Read the model definition and answer for the solid it produces. Units are mm, in the model's axes. A direction names the side the tool comes from. Give positions to 0.01 mm unless a question says otherwise; leave off trailing zeros. Order: outer loops, then holes, each group sorted by start corner. A loop starts at its lowest first (then second) coordinate and runs counter-clockwise, first axis right, second up. Notation, with made-up numbers: (-22.5, -9) - (11.5, -9) arc R28 ccw to (11.5, 16) - close; hole circle Ø11 at (-27, 21). An arc over 180 degrees is marked (long way). Return JSON: item names as keys, results as strings.
```python
from build123d import *

# Parameters (mm, degrees)
SKIZZE1_R                       = 30.405
SKIZZE1_R_2                     = 28.405
AUFSATZ_LINEAR_AUSTRAGEN1_DEPTH = 10
SKIZZE2_R                       = 30.405
AUFSATZ_LINEAR_AUSTRAGEN2_DEPTH = 1
AUFSATZ_LINEAR_START            = 10
AUFSATZ_LINEAR_AUSTRAGEN3_DEPTH = 10
SKIZZE5_R                       = 1.5
SCHNITT_LINEAR_AUSTRAGEN2_DEPTH = 10
SKIZZE6_W                       = 6
SKIZZE6_H                       = 10
SCHNITT_LINEAR_AUSTRAGEN3_DEPTH = 10


with BuildPart() as part:
    # Skizze1 → Aufsatz-Linear austragen1 (new body)
    with BuildSketch(Plane(origin=(0, 0, 0), x_dir=(1, 0, 0), z_dir=(0, 1, 0))):
        with Locations(Location((0, 0, 0), (0, 0, 270))):
            Circle(SKIZZE1_R)
        with Locations(Location((0, 0, 0), (0, 0, 270))):
            Circle(SKIZZE1_R_2, mode=Mode.SUBTRACT)
    extrude(amount=AUFSATZ_LINEAR_AUSTRAGEN1_DEPTH)

    # Skizze2 → Aufsatz-Linear austragen2 (add)
    with BuildSketch(Plane(origin=(0, 10, 0), x_dir=(1, 0, 0), z_dir=(0, 1, 0))):
        with Locations(Location((0, 0, 0), (0, 0, 270))):
            Circle(SKIZZE2_R)
    extrude(amount=AUFSATZ_LINEAR_AUSTRAGEN2_DEPTH)

    # Skizze4 → Aufsatz-Linear austragen3 (add)
    with BuildSketch(Plane.XZ.offset(-10).offset(AUFSATZ_LINEAR_START)):
        with BuildLine():
            ThreePointArc((-28.126789531, -3.965820935), (-23.605, 0), (-28.126789531, 3.965820935))
            ThreePointArc((-28.126789531, 3.965820935), (-28.405, 0), (-28.126789531, -3.965820935))
        make_face()
        with BuildLine():
            ThreePointArc((28.405, 0), (28.33536202, 1.987783738), (28.126789531, 3.965820935))
            ThreePointArc((28.126789531, 3.965820935), (23.605, 0), (28.126789531, -3.965820935))
            ThreePointArc((28.126789531, -3.965820935), (28.33536202, -1.987783738), (28.405, 0))
        make_face()
    extrude(amount=-AUFSATZ_LINEAR_AUSTRAGEN3_DEPTH)

    # Skizze5 → Schnitt-Linear austragen2 (cut)
    with BuildSketch(Plane.XZ):
        with Locations(Location((-27.605, 0, 0), (0, 0, 270))):
            Circle(SKIZZE5_R)
        with BuildLine():
            ThreePointArc((29.105, 0), (27.605, 1.5), (26.105, 0))
            Line((26.105, 0), (29.105, 0))
        make_face()
        with BuildLine():
            Line((29.105, 0), (26.105, 0))
            ThreePointArc((26.105, 0), (27.605, -1.5), (29.105, 0))
        make_face()
    extrude(amount=-SCHNITT_LINEAR_AUSTRAGEN2_DEPTH, mode=Mode.SUBTRACT)

    # Skizze6 → Schnitt-Linear austragen3 (cut)
    with BuildSketch(Plane(origin=(0, 11, 0), x_dir=(1, 0, 0), z_dir=(0, 1, 0))):
        with Locations((-7.328778972, -13.508309901)):
            Rectangle(SKIZZE6_W, SKIZZE6_H)
    extrude(amount=-SCHNITT_LINEAR_AUSTRAGEN3_DEPTH, mode=Mode.SUBTRACT)


solid = part.part
```
Q1. Consider L1, parallel to Z at x = 24, y = 5; L2, parallel to Z at x = -25.5, y = 3.75; L3, parallel to Y at x = -12.5, z = 12. Determine where each line is inside the solid, lowest interval first.
Values:
{"L1": "z = -18.67 to -15.19, -1.73 to 1.73, 15.19 to 18.67", "L2": "z = -16.56 to -12.51, -3.4 to 3.4, 12.51 to 16.56", "L3": "y = 10 to 11"}
Q2. Given pin 1 (1.8 mm diameter, centred on x = 27.605, z = 0, fed in from -Y); pin 2 (0.5 mm diameter, centred on x = -7, y = 10.5, fed in from +Z); pin 3 (0.8 mm diameter, centred on y = 10.5, z = 14, fed in from -X), each flat-ended and moving along its own axis, determine where each tip first touches the part or whether it passes through.
Values:
{"pin 1": "stops at y = 10", "pin 2": "stops at z = 29.65", "pin 3": "stops at x = -27.19"}
Q3. A cutting plane is placed at B-B (y = 7.25). Write down the section's boundary in (x, z) (3 decimals).
Values:
{"outline": "circle Ø60.81 at (0, 0); hole circle Ø3 at (-27.605, 0); hole (-28.127, -3.966) arc R28.405 ccw to (28.127, -3.966) arc R4 cw (long way) to (28.127, 3.966) arc R28.405 ccw to (-28.127, 3.966) arc R4 cw (long way) to start; hole circle Ø3 at (27.605, 0)"}
Q4. A cutting plane is placed at D-D (x = 19.5). Write down the section's boundary in (y, z), and give its area (3 significant figures).
Values:
{"outline": "(0, -23.33) - (11, -23.33) - (11, 23.33) - (0, 23.33) - (0, 20.65) - (10, 20.65) - (10, -20.65) - (0, -20.65) - close", "area": "100 mm²"}
Q5. A cutting plane is placed at A-A (z = 0). Write down the section's boundary in (x, y) (3 decimals), and give its area (3 significant figures).
Values:
{"outline": "(-30.405, 0) - (-29.105, 0) - (-29.105, 10) - (-26.105, 10) - (-26.105, 0) - (-23.605, 0) - (-23.605, 10) - (23.605, 10) - (23.605, 0) - (26.105, 0) - (26.105, 10) - (29.105, 10) - (29.105, 0) - (30.405, 0) - (30.405, 11) - (-30.405, 11) - close", "area": "137 mm²"}
Q6. For faces 1 (the flat face through (0, 10, 0)), 2 (the flat face through (25, 0, 0)), determine the directions among +Z, -Z, +X, -X, +Y, -Y from which every point of the face is accessible in a straight line to the end or side of a thin tool.
Values:
{"face 1": "-Y", "face 2": "+Z, -Z, +X, -X, -Y"}
Q7. A cutting plane is placed at C-C (x = 0). Write down the section's boundary in (y, z) (3 decimals), and give its area (3 significant figures).
Values:
{"outline": "(0, -30.405) - (11, -30.405) - (11, 30.405) - (0, 30.405) - (0, 28.405) - (10, 28.405) - (10, -28.405) - (0, -28.405) - close", "area": "101 mm²"}
